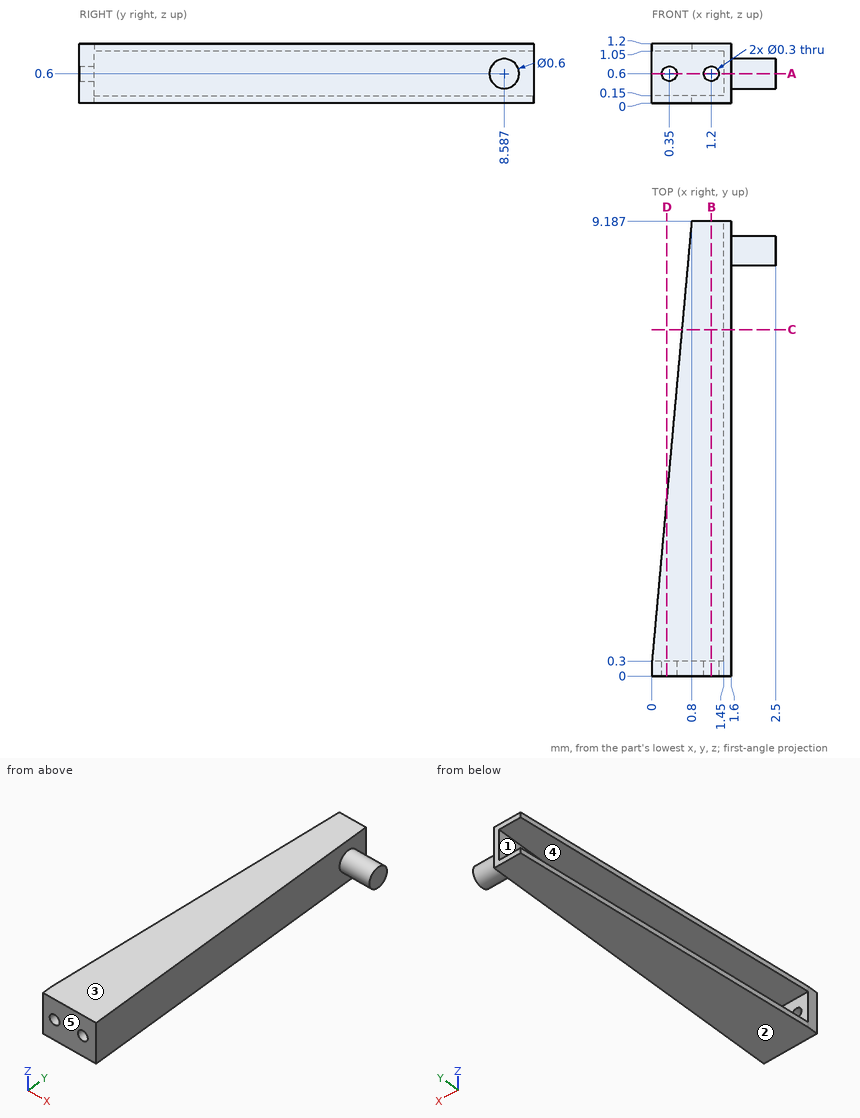
Geometry check sheet. Reference: drawing and pictorial views, mm from the part's lowest x, y, z. A direction names the side the tool comes from. Round coordinates to 2 decimals unless told otherwise and drop trailing zeros. Write each loop counter-clockwise with the first axis right and the second up, starting at its lowest first coordinate (ties: lowest second). Pieces come first, ordered by that corner, then holes. Notation, with made-up numbers: (73.25, 86.5) -> (127.25, 86.5) arc R31 ccw to (127.25, 110.5) -> close; hole circle Ø3 at (71, 15.25). An arc over 180 degrees is marked (long way). Answer as CSV lines item,"result". Start each with the question number.
1) Material ranges on line 1 (X direction, y = 0.1, z = 0.6); line 2 (Z direction, x = 1.2, y = 0.15); line 3 (Y direction, x = 0.1, z = 0.7), recorded low to high. Write a range as from..to.
2) Section check C-C on y = 7. Enter the section's corners in (x, z).
3) Section check B-B on x = 1.2. Enter the section's corners in (y, z), and give its area (3 significant figures).
4) Go/stop test with flat-tipped pins: P1, Ø0.5, axis at y = 3, z = 1, coming from the -X side; P2, Ø0.7, axis at x = 1, y = 6, coming from the -Z side. Record where each tip stops, or that it passes through.
5) Section check A-A on z = 0.6. Enter the section's corners in (x, y), and give its area (3 significant figures).
6) Tool access check on the marked faces 1 and 2. Record the directions out of +Z, -Z, +X, -X, +Y, -Y that give a thin tool (end or side, any length) a straight path to the whole face; none if there is none.
7) Release check for a two-part mould opening along Z. For the marked faces 3, 4 and 5 record: pulls with the +Z half, pulls with the -Z half, needs draft (parallel to the pull), parting line crosses it, or undercut.
8) Section check D-D on x = 0.3. Enter the section's corners in (y, z), and give its area (3 significant figures).
Found:
1,line 1,"x = 0..0.2, 0.5..1.05, 1.35..1.6"
1,line 2,"z = 0..0.45, 0.75..1.2"
1,line 3,"y = 0..0.3"
2,outline,"(0.6, 0) -> (1.6, 0) -> (1.6, 1.2) -> (0.6, 1.2) -> (0.6, 1.05) -> (1.45, 1.05) -> (1.45, 0.15) -> (0.6, 0.15) -> close"
3,outline,"(0, 0) -> (9.19, 0) -> (9.19, 0.15) -> (0.3, 0.15) -> (0.3, 0.45) -> (0, 0.45) -> close; (0, 0.75) -> (0.3, 0.75) -> (0.3, 1.05) -> (9.19, 1.05) -> (9.19, 1.2) -> (0, 1.2) -> close"
3,area,"2.94 mm^2"
4,P1,"stops at x = 0.22"
4,P2,"stops at z = 0"
5,outline,"(0, 0) -> (0.2, 0) -> (0.2, 0.3) -> (0, 0.3) -> close; (0.5, 0) -> (1.05, 0) -> (1.05, 0.3) -> (0.5, 0.3) -> close; (1.35, 0) -> (1.6, 0) -> (1.6, 8.29) -> (2.5, 8.29) -> (2.5, 8.89) -> (1.6, 8.89) -> (1.6, 9.19) -> (1.45, 9.19) -> (1.45, 0.3) -> (1.35, 0.3) -> close"
5,area,"2.17 mm^2"
6,face 1,"-X, +Y"
6,face 2,"-Z, +X, -X, +Y, -Y"
7,face 3,"pulls with the +Z half"
7,face 4,"undercut"
7,face 5,"needs draft"
8,outline,"(0, 0) -> (3.63, 0) -> (3.63, 0.15) -> (0.3, 0.15) -> (0.3, 0.46) -> (0, 0.46) -> close; (0, 0.74) -> (0.3, 0.74) -> (0.3, 1.05) -> (3.63, 1.05) -> (3.63, 1.2) -> (0, 1.2) -> close"
8,area,"1.27 mm^2"
